Input: part model. Units: mm. Frame: model coordinates. Face numbers are marked on the shaded views. Give positions to 0.01 mm unless a question says otherwise; leave off trailing zeros. Loops run counter-clockwise (first coordinate to the right, second up) from the corner with the lowest first, then second, coordinate; pieces in that order, holes last. Notation, with made-up numbers: (37, 16.25) - (78, 16.25) arc R21 ccw to (78, 48.25) - close; hole circle Ø1 at (36.5, 17.25). An arc over 180 degrees is marked (long way). Answer as a JSON object with one key per item and string values. Group by question number.
(1) Material intervals for L1, parallel to X at y = 19, z = 0; L2, parallel to X at y = 21.5, z = 3.75, sorted ascending.
(2) Section query B-B (x = 0). Return loops of the section in (y, z).
(3) Pin query (flat end, axial travel): P1, Ø1, axis at x = -4, z = -3, coming from the +Y side; P2, Ø3, axis at x = 16, y = 5, coming from the +Z side; P3, Ø5, axis at x = -17.5, z = -6, coming from the +Y side. Return the tip coordinate at first contact, or that it passes through.
(4) Section query A-A (z = 0). Return loops of the section in (x, y), plus the area to 3 significant figures.
(5) Section query C-C (y = 23.5). Return loops of the section in (x, z).
(6) Mould query, pull axis X, two halves, no side actions, for the marked faces 1, 2 and 3. Classes: +X half, -X half, draft (parallel to the pull), parting line (faces both ways), or undercut.
```python
from build123d import *

# Parameters (mm, degrees)
RUNROUTE_R           = 10.668
RUNEXTRUDE_DEPTH     = 25.4
OUTLETROUTE_R        = 10.668
OUTLETEXTRUDE_DEPTH  = 25.4
TEESHELL_START       = -25.4
TEESHELL_OUTLINE_R   = 7.8994
TEESHELL_DEPTH       = 50.8
TEESHELL_START_2     = -1e-07
TEESHELL_2_OUTLINE_R = 7.8994
TEESHELL_2_DEPTH     = 25.4000001
TEECHAMFER_SIZE      = 0.922866667


with BuildPart() as part:
    # RunRoute → RunExtrude (new body)
    with BuildSketch(Plane(origin=(0, 0, 0), x_dir=(0, 0, -1), z_dir=(1, 0, 0))):
        Circle(RUNROUTE_R)
    runextrude = extrude(amount=RUNEXTRUDE_DEPTH)

    # RunExtrudeMirror: RunExtrude across plane
    add(runextrude.mirror(Plane(origin=(0, 0, 0), x_dir=(0, 0, 1), z_dir=(1, 0, 0))))

    # OutletRoute → OutletExtrude (add)
    with BuildSketch(Plane(origin=(0, 0, 0), x_dir=(1, 0, 0), z_dir=(0, 1, 0))):
        with Locations(Location((0, 0, 0), (0, 0, 270))):
            Circle(OUTLETROUTE_R)
    extrude(amount=OUTLETEXTRUDE_DEPTH)

    # TeeShell: read off the stored shape, not the designer's step
    # TeeShell outline → TeeShell (cut)
    with BuildSketch(Plane.YZ.offset(TEESHELL_START)):
        Circle(TEESHELL_OUTLINE_R)
    extrude(amount=TEESHELL_DEPTH, mode=Mode.SUBTRACT)

    # TeeShell 2 outline → TeeShell 2 (cut)
    with BuildSketch(Plane(origin=(0, 0, 0), x_dir=(1, 0, 0), z_dir=(0, 1, 0)).offset(TEESHELL_START_2)):
        Circle(TEESHELL_2_OUTLINE_R)
    extrude(amount=TEESHELL_2_DEPTH, mode=Mode.SUBTRACT)

    # TeeChamfer
    # the kernel refuses this chamfer: 0.922866667 mm, written as the material it takes off along each edge
    with BuildSketch(Plane(origin=(25.4, 0, 0), x_dir=(0, 0, -1), z_dir=(0, -1, 0))) as teechamfer_piece_1:
        Polygon((10.668, -TEECHAMFER_SIZE), (10.668 - TEECHAMFER_SIZE, 0), (10.668, 0), align=None)
    revolve(axis=Axis((25.4, 0, 0), (1, 0, 0)), mode=Mode.SUBTRACT)
    with BuildSketch(Plane(origin=(-25.4, 0, 0), x_dir=(0, 0, -1), z_dir=(0, -1, 0))) as teechamfer_piece_2:
        Polygon((10.668, TEECHAMFER_SIZE), (10.668 - TEECHAMFER_SIZE, 0), (10.668, 0), align=None)
    revolve(axis=Axis((-25.4, 0, 0), (1, 0, 0)), mode=Mode.SUBTRACT)
    with BuildSketch(Plane(origin=(0, 25.4, 0), x_dir=(0, 0, 1), z_dir=(-1, 0, 0))) as teechamfer_piece_3:
        Polygon((10.668, -TEECHAMFER_SIZE), (10.668 - TEECHAMFER_SIZE, 0), (10.668, 0), align=None)
    revolve(axis=Axis((0, 25.4, 0), (0, 1, 0)), mode=Mode.SUBTRACT)


solid = part.part
```
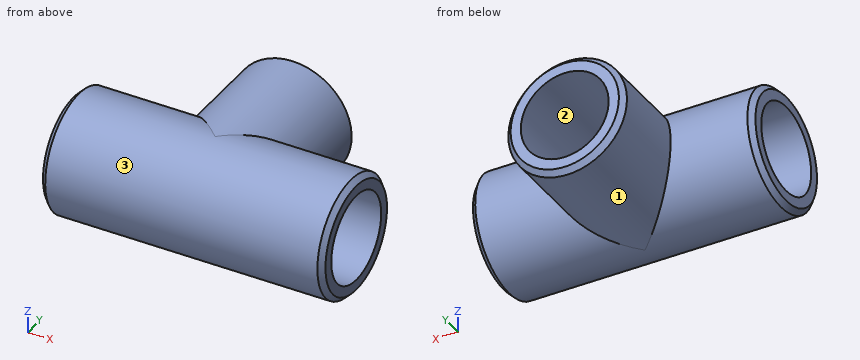
Recorded:
{
 "1": {"L1": "x = -10.67 to -7.9, 7.9 to 10.67", "L2": "x = -9.99 to -6.95, 6.95 to 9.99"},
 "2": {"outline": "(0, -10.67) - (24.48, -10.67) - (25.4, -9.75) - (25.4, -7.9) - (0, -7.9) arc R7.9 cw to (0, 7.9) - (25.4, 7.9) - (25.4, 9.75) - (24.48, 10.67) - (0, 10.67) arc R10.67 ccw to start"},
 "3": {"P1": "stops at y = -7.08", "P2": "stops at z = 10.08", "P3": "stops at y = 10.08"},
 "4": {"outline": "(-25.4, -9.75) - (-24.48, -10.67) - (24.48, -10.67) - (25.4, -9.75) - (25.4, -7.9) - (-25.4, -7.9) - close; (-25.4, 7.9) - (-7.9, 7.9) - (-7.9, 25.4) - (-9.75, 25.4) - (-10.67, 24.48) - (-10.67, 10.67) - (-24.48, 10.67) - (-25.4, 9.75) - close; (7.9, 7.9) - (25.4, 7.9) - (25.4, 9.75) - (24.48, 10.67) - (10.67, 10.67) - (10.67, 24.48) - (9.75, 25.4) - (7.9, 25.4) - close", "area": "317 mm^2"},
 "5": {"outline": "circle Ø21.34 at (0, 0); hole circle Ø15.8 at (0, 0)"},
 "6": {"face 1": "parting line", "face 2": "undercut", "face 3": "draft"}
}
